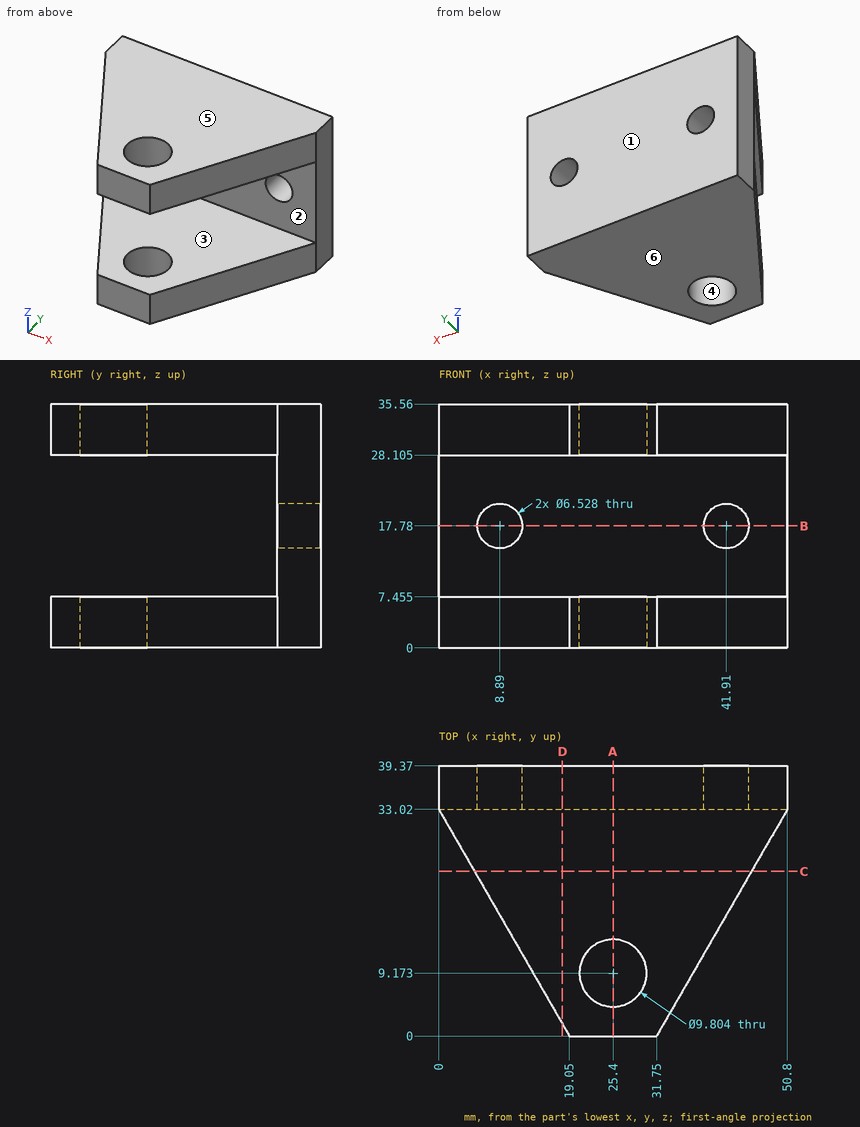
Verification items for this drawing (mm, ordinates from the low corner). A direction names the side the tool comes from. Coordinates: 2 decimals unless noted, no trailing zeros. Loops run counter-clockwise (first coordinate to the right, second up) from the corner with the lowest first, then second, coordinate; pieces in that order, holes last. Notation, with made-up numbers: (-31.5, 45) -> (-3.5, 45) arc R8 ccw to (-3.5, 50) -> close; hole circle Ø9 at (67.5, 46.5). An arc over 180 degrees is marked (long way). Put each result on its own line as item: value.
1. Gauge pin test, flat ends, axial feed: P1, Ø3, axis at x = 9.5, z = 9, coming from the -Y side; P2, Ø4, axis at x = 35, y = 23.5, coming from the -Z side; P3, Ø1, axis at x = 36.5, z = 4, coming from the -Y side (1 decimal); P4, Ø1.5, axis at y = 29.5, z = 30.5, coming from the -X side. Record the tip position at first contact, or that the pin passes through.
Result set:
P1: stops at y = 33.02
P2: stops at z = 0
P3: stops at y = 7.4
P4: stops at x = 1.6
2. Tool access check on the marked faces 1 and 2. Record the directions out of +Z, -Z, +X, -X, +Y, -Y that give a thin tool (end or side, any length) a straight path to the whole face; none if there is none.
Result set:
face 1: +Z, -Z, +X, -X, +Y
face 2: +X, -X, -Y
3. Section check B-B, the plane z = 17.78. Record the boundary of the cut face in (x, y).
Result set:
outline: (0, 33.02) -> (5.63, 33.02) -> (5.63, 39.37) -> (0, 39.37) -> close; (12.15, 33.02) -> (38.65, 33.02) -> (38.65, 39.37) -> (12.15, 39.37) -> close; (45.17, 33.02) -> (50.8, 33.02) -> (50.8, 39.37) -> (45.17, 39.37) -> close
4. Section check C-C, the plane y = 24. Record the boundary of the cut face in (x, z) (1 decimal), then the cut area to 3 significant figures.
Result set:
outline: (5.2, 0) -> (45.6, 0) -> (45.6, 7.5) -> (5.2, 7.5) -> close; (5.2, 28.1) -> (45.6, 28.1) -> (45.6, 35.6) -> (5.2, 35.6) -> close
area: 602 mm^2
5. Section check D-D, the plane x = 18. Record the boundary of the cut face in (y, z) (1 decimal).
Result set:
outline: (1.8, 0) -> (39.4, 0) -> (39.4, 35.6) -> (1.8, 35.6) -> (1.8, 28.1) -> (33, 28.1) -> (33, 7.5) -> (1.8, 7.5) -> close
6. Thickness scan on line 1 (X direction, y = 36, z = 17.78); line 2 (Y direction, x = 25.4, z = 34) (1 decimal); line 3 (Z direction, x = 32.5, y = 16) (1 decimal). Record the ranges inside material, lowest first.
Result set:
line 1: x = 0 to 5.63, 12.15 to 38.65, 45.17 to 50.8
line 2: y = 0 to 4.3, 14.1 to 39.4
line 3: z = 0 to 7.5, 28.1 to 35.6
7. Section check A-A, the plane x = 25.4. Record the boundary of the cut face in (y, z) (1 decimal), then the cut area to 3 significant figures.
Result set:
outline: (0, 0) -> (4.3, 0) -> (4.3, 7.5) -> (0, 7.5) -> close; (0, 28.1) -> (4.3, 28.1) -> (4.3, 35.6) -> (0, 35.6) -> close; (14.1, 0) -> (39.4, 0) -> (39.4, 35.6) -> (14.1, 35.6) -> (14.1, 28.1) -> (33, 28.1) -> (33, 7.5) -> (14.1, 7.5) -> close
area: 572 mm^2
8. Mould release check, pull along Z, two halves, no side actions. Record for the marked faces 3, 4, 5 and 6: pulls with the +Z half, pulls with the -Z half, needs draft (parallel to the pull), parting line crosses it, or undercut.
Result set:
face 3: undercut
face 4: needs draft
face 5: pulls with the +Z half
face 6: pulls with the -Z half
